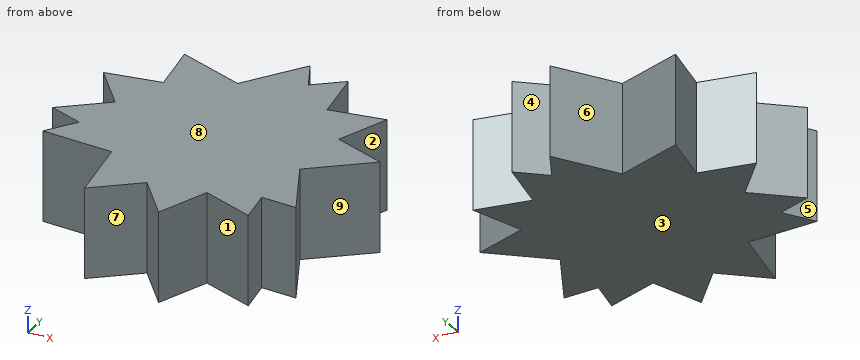
from build123d import *

# Parameters (mm, degrees)
F1_DEPTH = 25.4


with BuildPart() as f1:
    # F0 (on Top) → F1 (new body)
    with BuildSketch(Plane.XY):
        Polygon((27.8356494382, 12.1693564579), (33.5699106521, 26.8122048944), (18.0217013154, 24.4567965593), (19.3815969517, 15.4800337134), align=None)
        Polygon((42.4784978747, 6.435095244), (27.8356494382, 12.1693564579), (23.3848302984, 0.8038696669), (26.688019605, -6.1767208295), align=None)
        Polygon((23.3848302984, 0.8038696669), (27.8356494382, 12.1693564579), (19.3815969517, 15.4800337134), (20.7667316179, 6.3366663281), align=None)
        Polygon((19.3815969517, 15.4800337134), (18.0217013154, 24.4567965593), (12.5822778175, 23.6327747593), (15.7710654967, 16.8939478554), align=None)
        Polygon((12.5822778175, 23.6327747593), (18.0217013154, 24.4567965593), (15.6662929803, 40.0050058961), (7.8057995659, 33.7268491806), align=None)
        Polygon((26.688019605, -6.1767208295), (23.3848302984, 0.8038696669), (22.1013882243, -2.4734919786), (23.096900923, -9.0449384694), align=None)
        Polygon((2.4734919786, 22.1013882243), (12.5822778175, 23.6327747593), (7.8057995659, 33.7268491806), (-3.7153039714, 24.5249721827), align=None)
        Polygon((35.3318663109, -24.443658799), (26.688019605, -6.1767208295), (23.096900923, -9.0449384694), (25.3054083971, -23.6234453112), align=None)
        Polygon((-3.7153039714, 24.5249721827), (7.8057995659, 33.7268491806), (3.502896326, 42.8201231878), (-7.9948126521, 26.2008633694), align=None)
        Polygon((23.096900923, -9.0449384694), (17.9036176718, -13.1928010017), (14.1754443947, -22.7129596071), (25.3054083971, -23.6234453112), align=None)
        Polygon((-12.388586702, 19.8499222681), (-8.9085872226, 20.3771096504), (-3.7153039714, 24.5249721827), (-7.9948126521, 26.2008633694), align=None)
        Polygon((25.3054083971, -23.6234453112), (14.1754443947, -22.7129596071), (12.1693564579, -27.8356494382), (26.8122048944, -33.5699106521), align=None)
        Polygon((12.1693564579, -27.8356494382), (14.1754443947, -22.7129596071), (6.7450552646, -22.1051172926), (3.7153039714, -24.5249721827), align=None)
        Polygon((-15.8710798244, 14.8161839706), (-12.388586702, 19.8499222681), (-24.4567965593, 18.0217013154), (-23.096900923, 9.0449384694), align=None)
        Polygon((-24.4567965593, 18.0217013154), (-12.388586702, 19.8499222681), (-7.9948126521, 26.2008633694), (-26.8122048944, 33.5699106521), align=None)
        Polygon((6.435095244, -42.4784978747), (12.1693564579, -27.8356494382), (3.7153039714, -24.5249721827), (-3.3788528789, -30.1910577733), align=None)
        Polygon((3.7153039714, -24.5249721827), (-4.8956517935, -21.1528502987), (-10.9962435963, -20.653791935), (-3.3788528789, -30.1910577733), align=None)
        Polygon((-23.096900923, 9.0449384694), (-24.4567965593, 18.0217013154), (-40.0050058961, 15.6662929803), (-30.1910577733, 3.3788528789), align=None)
        Polygon((-26.7577222122, -0.9198151522), (-22.5161207613, 5.2111694372), (-23.096900923, 9.0449384694), (-30.1910577733, 3.3788528789), align=None)
        Polygon((-18.693206953, -20.0241425399), (-10.9962435963, -20.653791935), (-13.1928010017, -17.9036176718), (-19.3815969517, -15.4800337134), align=None)
        Polygon((-3.3788528789, -30.1910577733), (-10.9962435963, -20.653791935), (-18.693206953, -20.0241425399), (-15.6662929803, -40.0050058961), align=None)
        Polygon((-33.111207963, -10.1034038694), (-26.7577222122, -0.9198151522), (-30.1910577733, 3.3788528789), (-42.4784978747, -6.435095244), align=None)
        Polygon((-20.3771096504, -8.9085872226), (-26.7577222122, -0.9198151522), (-33.111207963, -10.1034038694), (-19.3815969517, -15.4800337134), align=None)
        Polygon((-38.8347626368, -18.3764643888), (-18.693206953, -20.0241425399), (-19.3815969517, -15.4800337134), (-33.111207963, -10.1034038694), align=None)
        Polygon((17.9036176718, -13.1928010017), (22.1013882243, -2.4734919786), (20.7667316179, 6.3366663281), (15.7710654967, 16.8939478554), (2.4734919786, 22.1013882243), (-8.9085872226, 20.3771096504), (-15.8710798244, 14.8161839706), (-22.5161207613, 5.2111694372), (-20.3771096504, -8.9085872226), (-13.1928010017, -17.9036176718), (-4.8956517935, -21.1528502987), (6.7450552646, -22.1051172926), align=None)
        Polygon((15.7710654967, 16.8939478554), (12.5822778175, 23.6327747593), (2.4734919786, 22.1013882243), align=None)
        Polygon((20.7667316179, 6.3366663281), (19.3815969517, 15.4800337134), (15.7710654967, 16.8939478554), align=None)
        Polygon((22.1013882243, -2.4734919786), (23.3848302984, 0.8038696669), (20.7667316179, 6.3366663281), align=None)
        Polygon((23.096900923, -9.0449384694), (22.1013882243, -2.4734919786), (17.9036176718, -13.1928010017), align=None)
        Polygon((14.1754443947, -22.7129596071), (17.9036176718, -13.1928010017), (6.7450552646, -22.1051172926), align=None)
        Polygon((3.7153039714, -24.5249721827), (6.7450552646, -22.1051172926), (-4.8956517935, -21.1528502987), align=None)
        Polygon((-10.9962435963, -20.653791935), (-4.8956517935, -21.1528502987), (-13.1928010017, -17.9036176718), align=None)
        Polygon((-19.3815969517, -15.4800337134), (-13.1928010017, -17.9036176718), (-20.3771096504, -8.9085872226), align=None)
        Polygon((-20.3771096504, -8.9085872226), (-22.5161207613, 5.2111694372), (-26.7577222122, -0.9198151522), align=None)
        Polygon((-22.5161207613, 5.2111694372), (-15.8710798244, 14.8161839706), (-23.096900923, 9.0449384694), align=None)
        Polygon((-15.8710798244, 14.8161839706), (-8.9085872226, 20.3771096504), (-12.388586702, 19.8499222681), align=None)
        Polygon((-8.9085872226, 20.3771096504), (2.4734919786, 22.1013882243), (-3.7153039714, 24.5249721827), align=None)
    extrude(amount=F1_DEPTH)


solid = f1.part
Geometry check sheet. Reference: the model listing, model coordinates, mm. Face numbers are marked on the shaded views. A direction names the side the tool comes from. Give positions to 0.01 mm unless a question says otherwise; leave off trailing zeros. Loops run counter-clockwise (first coordinate to the right, second up) from the corner with the lowest first, then second, coordinate; pieces in that order, holes last. Notation, with made-up numbers: M 42.25,55.25 L 75.25,55.25 A18 cw 75.25,75.25 Z; hole C -38,11 d8. An arc over 180 degrees is marked long. Answer as a JSON object with one key per item and string values. Group by question number.
Item 1: Mould release check, pull along X, two halves, no side actions. Record for the marked faces 1, 2, 3 and 4: pulls with the +X half, pulls with the -X half, needs draft (parallel to the pull), parting line crosses it, or undercut.
Item 2: Sectioned sample at C-C on y = 21. Record the boundary of the cut face in (x, z).
Item 3: Gauge pin test, flat ends, axial feed: pin 1 (2 mm diameter, centred on y = -22, z = 8.5, fed in from +X); pin 2 (1 mm diameter, centred on y = 3.5, z = 16.5, fed in from -X); pin 3 (1 mm diameter, centred on y = -3.5, z = 10, fed in from +X). Record the tip position at first contact, or that the pin passes through.
Item 4: Sectioned sample at A-A on y = -35. Record the boundary of the cut face in (x, z).
Item 5: Sectioned sample at D-D on y = -16.5. Record the boundary of the cut face in (x, z), plus the area to 3 significant figures.
Item 6: Sectioned sample at B-B on z = 5.75. Record the boundary of the cut face in (x, y) (1 decimal), plus the area to 3 significant figures.
Item 7: Access from +Z, -Z, +X, -X, +Y, -Y to the whole of each face (thin tool, end or side, straight path). Record for the marked faces 5, 6, 7, 8 and 9.
Item 8: Material ranges on L1, parallel to X at y = 35.5, z = 4.25; L2, parallel to X at y = -35.5, z = 8.5; L3, parallel to X at y = -23.5, z = 4.75, recorded low to high.
Findings below:
{
 "1": {"face 1": "undercut", "face 2": "pulls with the +X half", "face 3": "needs draft", "face 4": "undercut"},
 "2": {"outline": "M -24.91,0 L 31.29,0 L 31.29,25.4 L -24.91,25.4 Z"},
 "3": {"pin 1": "x = 34.65", "pin 2": "x = -30.69", "pin 3": "x = 30.67"},
 "4": {"outline": "M -16.42,0 L -9.4,0 L -9.4,25.4 L -16.42,25.4 Z; M 0.46,0 L 9.36,0 L 9.36,25.4 L 0.46,25.4 Z"},
 "5": {"outline": "M -37.54,0 L 31.57,0 L 31.57,25.4 L -37.54,25.4 Z", "area": "1,760 mm2"},
 "6": {"outline": "M -42.5,-6.4 L -33.1,-10.1 L -38.8,-18.4 L -18.7,-20 L -15.7,-40 L -3.4,-30.2 L 6.4,-42.5 L 12.2,-27.8 L 26.8,-33.6 L 25.3,-23.6 L 35.3,-24.4 L 26.7,-6.2 L 42.5,6.4 L 27.8,12.2 L 33.6,26.8 L 18,24.5 L 15.7,40 L 7.8,33.7 L 3.5,42.8 L -8,26.2 L -26.8,33.6 L -24.5,18 L -40,15.7 L -30.2,3.4 Z", "area": "3,980 mm2"},
 "7": {"face 5": "+Z, -Z, -X", "face 6": "+Z, -Z, +Y", "face 7": "+Z, -Z, -Y", "face 8": "+Z, +X, -X, +Y, -Y", "face 9": "+Z, -Z, +X"},
 "8": {"L1": "-1.56 to 6.97, 10.03 to 16.35", "L2": "-16.35 to -10.03, 0.86 to 9.17", "L3": "-18.17 to 34.89"}
}
